Work out the finished part from the listing and answer in its coordinate system (mm). Face numbers are marked on the shaded views. A direction names the side the tool comes from. Coordinates: 2 decimals unless noted, no trailing zeros. Order: outer loops, then holes, each group sorted by start corner. A loop starts at its lowest first (then second) coordinate and runs counter-clockwise, first axis right, second up. Notation, with made-up numbers: (-0.5, -4.75) -> (9.5, -4.75) arc R20 ccw to (9.5, 16.25) -> close; hole circle Ø9 at (-0.75, 29.5). An arc over 180 degrees is marked (long way). Write item = value, one per line. Start each with the question number.
Q1. Straight lines are drawn through the part: L1, parallel to Z at x = -22.5, y = 2; L2, parallel to Y at x = -20, z = -1; L3, parallel to Z at x = -34.5, y = -9. For each, find the intervals that lie inside material, in ascending order. Write a range as from..to.
Q2. For a pull along Y with two mould halves and no side action, classify the marked faces 1, 2 and 3 as +Y half, -Y half, draft (parallel to the pull), parting line (faces both ways), or undercut.
Q3. The part is cut by section A-A, the plane z = -39. Determine the outline of the cut face in (x, y).
Q4. Which of the six approach directions +Z, -Z, +X, -X, +Y, -Y give full straight-line access (tool end or side, diameter ignored) to the marked faces 4, 5, 6, 7 and 8?
Q5. Flat-ended cylindrical pins translate along their axes: pin 1 (5.5 mm diameter, centred on x = -54, z = 0.5, fed in from -Y); pin 2 (1 mm diameter, centred on y = 5.5, z = -28.5, fed in from -X); pin 3 (15 mm diameter, centred on x = -44, z = 22, fed in from -Y); pin 4 (3 mm diameter, centred on y = -7, z = -7, fed in from -X). Find the tip coordinate at first contact, or state that the pin passes through.
Q6. The part is cut by section C-C, the plane x = -52. Determine the outline of the cut face in (y, z), plus the area to 3 significant figures.
Q7. The part is cut by section D-D, the plane z = 34.5. Determine the outline of the cut face in (x, y), plus the area to 3 significant figures.
Q8. The part is cut by section B-B, the plane x = 4.5. Determine the outline of the cut face in (y, z), plus the area to 3 significant figures.
```python
from build123d import *

# Parameters (mm, degrees)
SALIENTE_EXTRUIR2_DEPTH   = 46.49999999999997
CROQUIS3_R                = 1.5007742960379549
CROQUIS3_R_2              = 1.503322104684281
CORTAR_EXTRUIR1_DEPTH     = 46.49999999999997
CORTAR_EXTRUIR2_START     = 16.5
CORTAR_EXTRUIR2_OUTLINE_R = 1.500774296
CORTAR_EXTRUIR2_DEPTH     = 30
REDONDEO2_R               = 3
CORTAR_EXTRUIR3_START     = -46.5
CORTAR_EXTRUIR3_OUTLINE_R = 1.500774296
CORTAR_EXTRUIR3_DEPTH     = 30
REDONDEO3_R               = 3
CORTAR_EXTRUIR4_START     = 10
CORTAR_EXTRUIR4_OUTLINE_R = 1.503322105
CORTAR_EXTRUIR4_DEPTH     = 20
CORTAR_EXTRUIR5_START     = -30
CORTAR_EXTRUIR5_OUTLINE_R = 1.503322105
CORTAR_EXTRUIR5_DEPTH     = 20
REDONDEO4_R               = 1
CORTAR_EXTRUIR12_DEPTH    = 155.46083657878992
CROQUIS6_W                = 18.599999999999966
CROQUIS6_H                = 6.000000000000004
CORTAR_EXTRUIR13_DEPTH    = 133.823646460648
CROQUIS7_W                = 18.599999999999966
CROQUIS7_H                = 6.000000000000004
CORTAR_EXTRUIR14_DEPTH    = 133.823646460648
REDONDEO5_R               = 1.5
REDONDEO6_R               = 2


# Read off the part's stored shape, not the designer's step: Cortar-Extruir2, Cortar-Extruir3, Cortar-Extruir4, Cortar-Extruir5
with BuildPart() as part:
    # Croquis1 → Saliente-Extruir2 (new, symmetric)
    with BuildSketch(Plane.XY):
        with BuildLine():
            Line((-10.683677010448408, -0.13792021644576552), (-8.74048031278475, -4.500000000012256))
            Line((-8.74048031278475, -4.500000000012256), (39.00000000000001, -4.500000000012256))
            Line((39.00000000000001, -4.500000000012256), (39.00000000000001, -10.500000000012262))
            Line((39.00000000000001, -10.500000000012262), (-25.99999999999999, -10.500000000012262))
            Line((-25.99999999999999, -10.500000000012262), (-25.99999999999999, -26.10000000001226))
            Line((-25.99999999999999, -26.10000000001226), (-29.999999999999986, -26.100000000012262))
            Line((-29.999999999999986, -26.100000000012262), (-29.999999999999993, -10.500000000012264))
            Line((-29.999999999999993, -10.500000000012264), (-81.19999999999999, -10.500000000012271))
            ThreePointArc((-81.19999999999999, -10.500000000012271), (-82.6497474683058, -7.000000000012269), (-81.19999999999999, -3.5000000000122697))
            Line((-81.19999999999999, -3.5000000000122697), (-68.49110633124283, 8.777732226211745))
            ThreePointArc((-68.49110633124283, 8.777732226211745), (-65.27231144406849, 9.67090124633749), (-62.77037609438549, 7.457598074555828))
            Line((-62.77037609438549, 7.457598074555828), (-58.782136556190004, -3.5000000000122684))
            Line((-58.782136556190004, -3.5000000000122684), (-29.179236040573016, -3.500000000012267))
            Line((-29.179236040573016, -3.500000000012267), (-22.77115447929422, -2.1379202164457745))
            ThreePointArc((-22.77115447929422, -2.1379202164457745), (-21.470497358111732, 3.17610414183578), (-16.57695737694327, 0.729917256089285))
            ThreePointArc((-16.57695737694327, 0.729917256089285), (-13.63855195060632, 0.24007822050397465), (-10.683677010448408, -0.13792021644576552))
        make_face()
    extrude(amount=SALIENTE_EXTRUIR2_DEPTH, both=True)

    # Croquis3 → Cortar-Extruir1 (cut, symmetric)
    with BuildSketch(Plane.XY):
        with Locations((-66.05930026713617, 6.260527572915973)):
            Circle(CROQUIS3_R)
        with Locations((-19.999999999999996, 0)):
            Circle(CROQUIS3_R_2)
    extrude(amount=CORTAR_EXTRUIR1_DEPTH, both=True, mode=Mode.SUBTRACT)

    # Cortar-Extruir2 outline → Cortar-Extruir2 (cut)
    with BuildSketch(Plane.XY.offset(CORTAR_EXTRUIR2_START)):
        with BuildLine():
            Line((-68.491106331, 8.777732226), (-69.201699105, 8.091246996))
            ThreePointArc((-69.201699105, 8.091246996), (-66.848168988, 2.721235528), (-62.462991688, 6.61306636))
            Line((-62.462991688, 6.61306636), (-62.770376094, 7.457598075))
            ThreePointArc((-62.770376094, 7.457598075), (-65.272311444, 9.670901246), (-68.491106331, 8.777732226))
        make_face()
        with Locations((-66.059300267, 6.260527573)):
            Circle(CORTAR_EXTRUIR2_OUTLINE_R, mode=Mode.SUBTRACT)
    extrude(amount=CORTAR_EXTRUIR2_DEPTH, mode=Mode.SUBTRACT)

    # Redondeo2
    redondeo2_edges = [part.edges().sort_by_distance(p)[0] for p in [
        (-62.462991687999995, 6.613066360000001, 31.5),
    ]]
    fillet(redondeo2_edges, radius=REDONDEO2_R)

    # Cortar-Extruir3 outline → Cortar-Extruir3 (cut)
    with BuildSketch(Plane.XY.offset(CORTAR_EXTRUIR3_START)):
        with BuildLine():
            ThreePointArc((-69.164573514, 8.127113066), (-66.827048097, 2.685630168), (-62.508602445, 6.738380883))
            Line((-62.508602445, 6.738380883), (-62.770376094, 7.457598075))
            ThreePointArc((-62.770376094, 7.457598075), (-65.272311444, 9.670901246), (-68.491106331, 8.777732226))
            Line((-68.491106331, 8.777732226), (-69.164573514, 8.127113066))
        make_face()
        with Locations((-66.059300267, 6.260527573)):
            Circle(CORTAR_EXTRUIR3_OUTLINE_R, mode=Mode.SUBTRACT)
    extrude(amount=CORTAR_EXTRUIR3_DEPTH, mode=Mode.SUBTRACT)

    # Redondeo3
    redondeo3_edges = [part.edges().sort_by_distance(p)[0] for p in [
        (-62.508602444999994, 6.738380883, -31.5),
    ]]
    fillet(redondeo3_edges, radius=REDONDEO3_R)

    # Cortar-Extruir4 outline → Cortar-Extruir4 (cut)
    with BuildSketch(Plane.XY.offset(CORTAR_EXTRUIR4_START)):
        with BuildLine():
            Line((-22.771154479, -2.137920216), (-22.827271519, -2.149848262))
            ThreePointArc((-22.827271519, -2.149848262), (-18.523452571, -3.240720775), (-16.513304708, 0.718087877))
            ThreePointArc((-16.513304708, 0.718087877), (-16.545132262, 0.723996005), (-16.576957377, 0.729917256))
            ThreePointArc((-16.576957377, 0.729917256), (-21.470497358, 3.176104142), (-22.771154479, -2.137920216))
        make_face()
        with Locations((-20, 0)):
            Circle(CORTAR_EXTRUIR4_OUTLINE_R, mode=Mode.SUBTRACT)
    extrude(amount=CORTAR_EXTRUIR4_DEPTH, mode=Mode.SUBTRACT)

    # Cortar-Extruir5 outline → Cortar-Extruir5 (cut)
    with BuildSketch(Plane.XY.offset(CORTAR_EXTRUIR5_START)):
        with BuildLine():
            ThreePointArc((-22.813751372, -2.146974465), (-18.533466696, -3.203987987), (-16.523253553, 0.719933216))
            ThreePointArc((-16.523253553, 0.719933216), (-16.550106333, 0.724920565), (-16.576957377, 0.729917256))
            ThreePointArc((-16.576957377, 0.729917256), (-21.470497358, 3.176104142), (-22.771154479, -2.137920216))
            Line((-22.771154479, -2.137920216), (-22.813751372, -2.146974465))
        make_face()
        with Locations((-20, 0)):
            Circle(CORTAR_EXTRUIR5_OUTLINE_R, mode=Mode.SUBTRACT)
    extrude(amount=CORTAR_EXTRUIR5_DEPTH, mode=Mode.SUBTRACT)

    # Redondeo4
    redondeo4_edges = [part.edges().sort_by_distance(p)[0] for p in [
        (-69.20169910499999, 8.091246995999999, 31.5),
        (-69.164573514, 8.127113066, -31.5),
    ]]
    fillet(redondeo4_edges, radius=REDONDEO4_R)

    # Croquis3D6 → Cortar-Extruir12 (cut, through all)
    with BuildSketch(Plane(origin=(39.00000000000001, -10.500000000012262, -46.49999999999997), x_dir=(0, 0.30700277992275854, 0.9517086177605509), z_dir=(-1, 0, 0))):
        Polygon((0, 0), (17.701780290346246, -5.710251706563308), (19.543796969882806, 8.7e-16), (1.8420166795365527, 5.71025170656331), align=None)
    extrude(amount=CORTAR_EXTRUIR12_DEPTH, mode=Mode.SUBTRACT)

    # Croquis6 → Cortar-Extruir13 (cut, through all)
    with BuildSketch(Plane(origin=(39.00000000000001, 0, 0), x_dir=(0, 0, -1), z_dir=(1, 0, 0))):
        with Locations((-1.865e-14, -7.50000000001226)):
            Rectangle(CROQUIS6_W, CROQUIS6_H)
    extrude(amount=-CORTAR_EXTRUIR13_DEPTH, mode=Mode.SUBTRACT)

    # Croquis7 → Cortar-Extruir14 (cut, through all)
    with BuildSketch(Plane(origin=(39.00000000000001, 0, 0), x_dir=(0, 0, -1), z_dir=(1, 0, 0))):
        with Locations((-37.19999999999999, -7.50000000001226)):
            Rectangle(CROQUIS7_W, CROQUIS7_H)
    extrude(amount=-CORTAR_EXTRUIR14_DEPTH, mode=Mode.SUBTRACT)

    # Redondeo5
    redondeo5_edges = [part.edges().sort_by_distance(p)[0] for p in [
        (39.00000000000001, -7.500000000012258, -27.899999999999963),
        (15.12975984360763, -4.500000000012255, -27.899999999999963),
        (6.500000000000007, -10.50000000001226, -27.89999999999997),
        (39.00000000000001, -4.500000000012256, -18.599999999999966),
        (39.00000000000001, -10.500000000012262, -18.599999999999966),
        (6.500000000000007, -10.500000000012262, -9.299999999999965),
        (15.12975984360763, -4.500000000012258, -9.299999999999965),
        (6.500000000000007, -10.500000000012262, 9.300000000000002),
        (15.12975984360763, -4.500000000012258, 9.300000000000002),
        (39.00000000000001, -7.50000000001226, -9.299999999999965),
        (39.00000000000001, -7.50000000001226, 9.300000000000002),
        (39.00000000000001, -4.500000000012256, 18.600000000000005),
        (39.00000000000001, -10.500000000012262, 18.600000000000005),
        (15.12975984360763, -4.500000000012258, 27.900000000000006),
        (6.500000000000007, -10.500000000012262, 27.900000000000006),
        (39.00000000000001, -7.50000000001226, 27.900000000000006),
    ]]
    fillet(redondeo5_edges, radius=REDONDEO5_R)

    # Redondeo6
    redondeo6_edges = [part.edges().sort_by_distance(p)[0] for p in [
        (-10.683677010448406, -0.13792021644577176, 0),
    ]]
    fillet(redondeo6_edges, radius=REDONDEO6_R)


solid = part.part
```
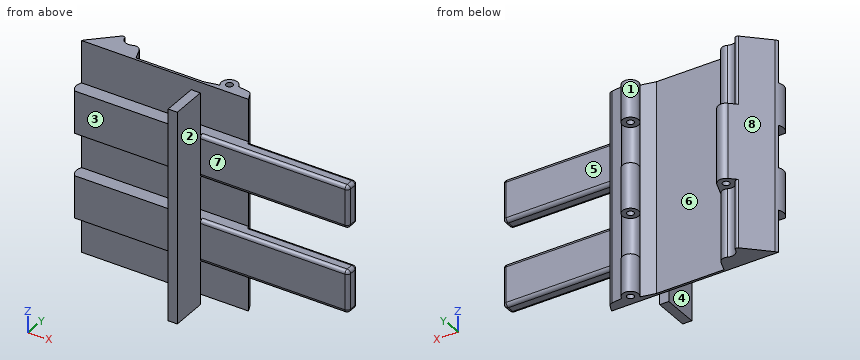
Model answer:
q1.L1 = -46.5..-30, -10..10, 30..46.5
q1.L2 = -4.5..-1.5, 1.5..3.5
q1.L3 = -27.9..-9.3, 9.3..27.9
q2.face_1 = undercut
q2.face_2 = draft
q2.face_3 = -Y half
q3.outline = (-81.97, -4.5) -> (-8.74, -4.5) -> (-10.22, -1.18) arc R2 ccw to (-11.8, -0.01) arc R78.5 cw to (-16.58, 0.73) arc R3.5 ccw (long way) to (-22.77, -2.14) -> (-29.18, -3.5) -> (-58.78, -3.5) -> (-60.51, 1.24) arc R3 ccw to (-64.58, 2.94) arc R3.62 cw to (-69.64, 5.53) arc R1 ccw to (-71.31, 6.05) -> (-81.2, -3.5) arc R4.95 ccw to start; (-30, -26.1) -> (-26, -26.1) -> (-26, -10.5) -> (-30, -10.5) -> close; hole circle Ø3.01 at (-20, 0)
q4.face_4 = +Z, -Z, -X, -Y
q4.face_5 = +Z, -Z, +X, +Y
q4.face_6 = +Z, -Z, +Y
q4.face_7 = +Z, -Z, +X, -Y
q4.face_8 = +Z, -Z, -X, +Y
q5.pin_1 = -4.5
q5.pin_2 = -72.4
q5.pin_3 = -10.5
q5.pin_4 = through
q6.outline = (-10.5, -27.9) -> (-4.5, -27.9) -> (-4.5, -46.5) -> (-3.5, -46.5) -> (-3.5, 46.5) -> (-4.5, 46.5) -> (-4.5, 27.9) -> (-10.5, 27.9) -> (-10.5, 9.3) -> (-4.5, 9.3) -> (-4.5, -9.3) -> (-10.5, -9.3) -> close
q6.area = 316 mm2
q7.outline = (-81.97, -4.5) -> (-8.74, -4.5) -> (-10.22, -1.18) arc R2 ccw to (-11.8, -0.01) arc R78.5 cw to (-16.58, 0.73) arc R3.5 ccw (long way) to (-22.77, -2.14) -> (-29.18, -3.5) -> (-58.78, -3.5) -> (-60.51, 1.26) arc R3 ccw to (-64.57, 2.96) arc R3.63 cw to (-69.62, 5.54) arc R1 ccw to (-71.3, 6.06) -> (-81.2, -3.5) arc R4.95 ccw to start; (-30, -26.1) -> (-26, -26.1) -> (-26, -10.5) -> (-30, -10.5) -> close; hole circle Ø3.01 at (-20, 0)
q7.area = 326 mm2
q8.outline = (-10.5, -26.4) arc R1.5 ccw to (-9, -27.9) -> (-6, -27.9) arc R1.5 ccw to (-4.5, -26.4) -> (-4.5, -10.8) arc R1.5 ccw to (-6, -9.3) -> (-9, -9.3) arc R1.5 ccw to (-10.5, -10.8) -> close; (-10.5, 10.8) arc R1.5 ccw to (-9, 9.3) -> (-6, 9.3) arc R1.5 ccw to (-4.5, 10.8) -> (-4.5, 26.4) arc R1.5 ccw to (-6, 27.9) -> (-9, 27.9) arc R1.5 ccw to (-10.5, 26.4) -> close
q8.area = 219 mm2
